Verification items for the finished model (mm, model axes). A direction names the side the tool comes from. Give positions to 0.01 mm unless a question says otherwise; leave off trailing zeros. Write each loop counter-clockwise with the first axis right and the second up, starting at its lowest first coordinate (ties: lowest second). Pieces come first, ordered by that corner, then holes. Notation, with made-up numbers: M -14,-16.75 L 17,-16.75 A22 ccw 17,-5.75 Z; hole C 76,-34 d6. An arc over 180 degrees is marked long. Write item = value, one per line.
from build123d import *
from OCP.BRepFilletAPI import BRepFilletAPI_MakeChamfer

# Parameters (mm, degrees)
BOSS_EXTRUDE1_DEPTH = 10
CHAMFER1_SIZE       = 1
CHAMFER1_SIZE2      = 0.866089989
CHAMFER2_SIZE       = 1
CHAMFER2_SIZE2      = 2.862737549


with BuildPart() as part:
    # Sketch1 → Boss-Extrude1 (new body)
    with BuildSketch(Plane(origin=(0, 0, 0), x_dir=(1, 0, 0), z_dir=(0, 1, 0))):
        Polygon((0, 0), (0, 45), (0, 47.5), (-2.5, 47.5), (-2.5, 45), (-5, 45), (-5, 50), (5, 50), (5, -50), (-5, -50), (-45, -26.25), (-45, -21.25), (-42.004108019, -21.25), (-42.004108019, -23.75), (-5, -23.75), (-5, -21.25), (-5, -2.5), (0, -2.5), align=None)
        Polygon((-37.793581703, -26.25), (-5, -45.721189136), (0, -45.721189136), (0, -26.25), align=None, mode=Mode.SUBTRACT)
    extrude(amount=BOSS_EXTRUDE1_DEPTH)

    # Chamfer1
    chamfer1_edges = [part.edges().sort_by_distance(p)[0] for p in [
        (-37.793581703, 5, 26.25),
    ]]
    chamfer1_side = [part.faces().sort_by_distance(p)[0] for p in [
        (-21.396790851, 5, 35.985594568),
    ]]
    chamfer(chamfer1_edges, length=CHAMFER1_SIZE, length2=CHAMFER1_SIZE2, reference=chamfer1_side[0])

    # Chamfer2: one chamfer whose edges measure the first distance from different faces: ONE call of the kernel's chamfer builder (chamfer() names one face for all edges)
    chamfer2_edges_1 = [part.edges().sort_by_distance(p)[0] for p in [
        (5, 5, 50),
        (-45, 5, 21.25),
        (-42.004108019, 5, 21.25),
        (-5, 5, 23.75),
        (-5, 5, 2.5),
        (0, 5, 2.5),
        (-2.5, 5, -45),
        (-5, 5, -45),
        (-5, 5, -50),
        (5, 5, -50),
        (0, 5, 45.721189136),
        (0, 5, 26.25),
    ]]
    chamfer2_edges_2 = [part.edges().sort_by_distance(p)[0] for p in [
        (-45, 5, 26.25),
    ]]
    chamfer2_side_2 = [part.faces().sort_by_distance(p)[0] for p in [
        (-45, 5, 23.75),
    ]]
    chamfer2 = BRepFilletAPI_MakeChamfer(part.part.solid().wrapped)
    for e in chamfer2_edges_1:
        chamfer2.Add(CHAMFER2_SIZE, e.wrapped)
    for e in chamfer2_edges_2:
        chamfer2.Add(CHAMFER2_SIZE, CHAMFER2_SIZE2, e.wrapped, chamfer2_side_2[0].wrapped)  # the first distance lies on this face
    add(Compound.cast(chamfer2.Shape()), mode=Mode.REPLACE)


solid = part.part
1) Cross-section at C-C on x = -36. Record the boundary of the cut face in (y, z), plus the area to 3 significant figures.
From the geometry:
outline = M 0,23.75 L 10,23.75 L 10,26.25 L 0,26.25 Z; M 0,27.31 L 10,27.31 L 10,31.59 L 0,31.59 Z
area = 67.8 mm^2
2) Depth check by flat-ended pin: P1, Ø3, axis at y = 6, z = 37.5, coming from the -X side; P2, Ø1.5, axis at x = -23.5, y = 1.5, coming from the +Z side; P3, Ø5, axis at y = 6.5, z = -28.5, coming from the -X side. Enter the tip coordinate at first touch or a pass-through.
From the geometry:
P1 = -28.58
P2 = 39.46
P3 = 0
3) Tool access check on faces 5 (the flat face through (-5, 5, -47)), 6 (the flat face through (-3, 5, 2.5)), 7 (the flat face through (-19, 5, 26.25)). Record the directions out of +Z, -Z, +X, -X, +Y, -Y that give a thin tool (end or side, any length) a straight path to the whole face; none if there is none.
From the geometry:
face_5 = -Z, -X, +Y, -Y
face_6 = -X, +Y, -Y
face_7 = +Y, -Y
4) Cross-section at B-B on z = 43. Record the boundary of the cut face in (x, y), plus the area to 3 significant figures.
From the geometry:
outline = M -16.79,0 L -9.58,0 L -9.58,10 L -16.79,10 Z; M 0,0 L 5,0 L 5,10 L 0,10 Z
area = 122 mm^2
5) Cross-section at D-D on z = -14. Record the boundary of the cut face in (x, y), plus the area to 3 significant figures.
From the geometry:
outline = M 0,0 L 5,0 L 5,10 L 0,10 Z
area = 50.0 mm^2
6) Draft check along Z on faces 1 (the flat face through (0, 5, -50)), 2 (the flat face through (0, 5, 36)), 3 (the flat face through (-5, 5, 13)), 4 (the flat face through (-1, 5, -47.5)). Enter one of: +Z half, -Z half, draft (parallel to the pull), parting line (faces both ways), or undercut.
From the geometry:
face_1 = -Z half
face_2 = undercut
face_3 = draft
face_4 = undercut
7) Material ranges on probe 1 along Z at (x, y) = (-0.5, 5.25); probe 2 along X at (y, z) = (9, -37.5); probe 3 along Z at (x, y) = (-10.5, 6), recorded low to high. Write a range as from..to.
From the geometry:
probe_1 = -50..-47.5, 2..26.75, 45.22..50
probe_2 = 0..5
probe_3 = 23.75..26.25, 42.46..46.73
